Could you check a few things on this drawing? It's one solid part, dimensions in mm from its lowest x, y, z. A direction names the side the tool comes from. Coordinates: 2 decimals unless noted, no trailing zeros. Loops run counter-clockwise (first coordinate to the right, second up) from the corner with the lowest first, then second, coordinate; pieces in that order, holes last. Notation, with made-up numbers: M 6.25,38.5 L 64.25,38.5 A16 ccw 64.25,67.5 Z; hole C 18,41 d10. An arc over 180 degrees is marked long. Use one line per item in the form item = value. Start each with the question number.
(1) On a 3-axis mill with a long thin cutter (end or side, diameter ignored), from which of +Z, -Z, +X, -X, +Y, -Y can I reach the whole of each face in a straight line? I mean the marked faces 1, 2 and 3. Say none if no direction works.
(2) Imagine slicing it at D-D, the plane x = 18. Please give me the cut outline in (y, z) (1 decimal).
(3) Thinking about a two-plate mould opening in Z: for the marked faces 4, 5 and 6, which applies, +Z half, -Z half, draft (parallel to the pull), parting line (faces both ways), or undercut?
(4) Imagine slicing it at C-C, the plane x = 27. Please give me the cut outline in (y, z) (1 decimal).
(5) Imagine slicing it at B-B, the plane y = 79.5. Please give me the cut outline in (x, z) (1 decimal), and give its area (3 significant figures).
(6) Please list where these lines run through material, in increasing order: L1, parallel to Z at x = 9, y = 62 (1 decimal); L2, parallel to Z at x = 9, y = 31 (1 decimal); L3, parallel to Y at x = 25.5, z = 67.5 (1 decimal).
(7) Will these pins go through, and if not, where does the flat tip stop? P1, Ø12.5, axis at x = 29.5, y = 30.5, coming from the -Z side; P2, Ø8, axis at y = 84.5, z = 82, coming from the -X side; P3, Ø4, axis at x = 3, z = 18.5, coming from the -Y side; P4, Ø3, axis at x = 2.5, z = 27.5, coming from the +Y side.
(8) Imagine slicing it at A-A, the plane z = 81. Please give me the cut outline in (x, y) (1 decimal), and give its area (3 significant figures).
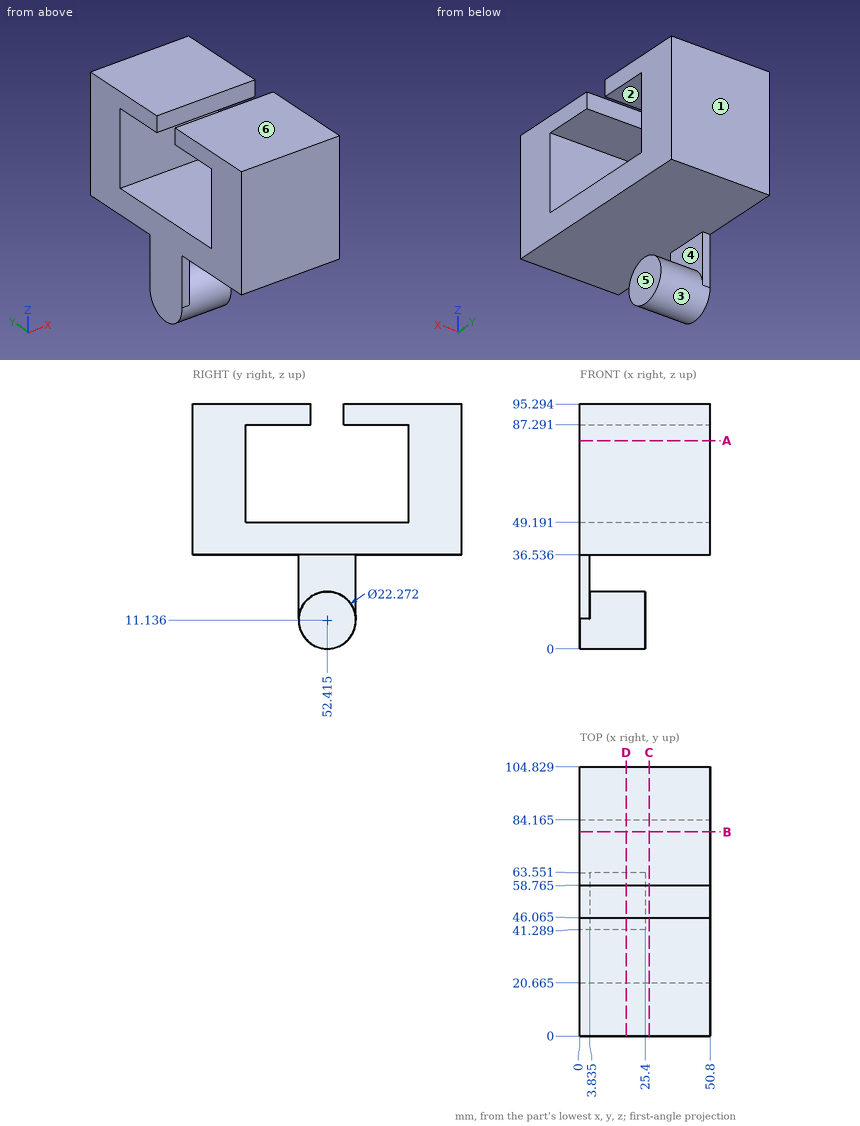
Answer:
q1.face_1 = +Z, -Z, +X, -X, +Y
q1.face_2 = +X, -X
q1.face_3 = +X
q2.outline = M 0,36.5 L 104.8,36.5 L 104.8,95.3 L 58.8,95.3 L 58.8,87.3 L 84.2,87.3 L 84.2,49.2 L 20.7,49.2 L 20.7,87.3 L 46.1,87.3 L 46.1,95.3 L 0,95.3 Z; C 52.4,11.1 d22.3
q3.face_4 = undercut
q3.face_5 = draft
q3.face_6 = +Z half
q4.outline = M 0,36.5 L 104.8,36.5 L 104.8,95.3 L 58.8,95.3 L 58.8,87.3 L 84.2,87.3 L 84.2,49.2 L 20.7,49.2 L 20.7,87.3 L 46.1,87.3 L 46.1,95.3 L 0,95.3 Z
q5.outline = M 0,36.5 L 50.8,36.5 L 50.8,49.2 L 0,49.2 Z; M 0,87.3 L 50.8,87.3 L 50.8,95.3 L 0,95.3 Z
q5.area = 1,050 mm²
q6.L1 = 5.5 to 16.8, 36.5 to 49.2, 87.3 to 95.3
q6.L2 = 36.5 to 49.2, 87.3 to 95.3
q6.L3 = 0 to 20.7, 84.2 to 104.8
q7.P1 = 36.54
q7.P2 = 0
q7.P3 = 41.29
q7.P4 = 63.55
q8.outline = M 0,0 L 50.8,0 L 50.8,20.7 L 0,20.7 Z; M 0,84.2 L 50.8,84.2 L 50.8,104.8 L 0,104.8 Z
q8.area = 2,100 mm²
